Here's how the part is built. I have some questions about the finished solid (model axes, mm). Face numbers are marked on the shaded views. A direction names the side the tool comes from. Coordinates: 2 decimals unless noted, no trailing zeros. Write each loop counter-clockwise with the first axis right and the second up, starting at its lowest first coordinate (ties: lowest second). Pieces come first, ordered by that corner, then holes.
(1) Imagine slicing it at B-B, the plane y = -1. List the corners of the cut face in (x, z) for me, plus the area to 3 significant figures.
(2) Please list where these lines run through material, in increasing order: probe 1 along Z at (x, y) = (1.25, -2.25); probe 2 along X at (y, z) = (-1, -1); probe 3 along Y at (x, z) = (2.5, -32.5).
(3) Imagine slicing it at C-C, the plane z = -30. List the corners of the cut face in (x, y) for me.
(4) Imagine slicing it at A-A, the plane x = 0. List the corners of the cut face in (y, z) for me.
(5) Imagine slicing it at D-D, the plane x = -2.25. List the corners of the cut face in (y, z) for me.
(6) Which directions (+Z, -Z, +X, -X, +Y, -Y) give clear straight access to the entire face, cutting with the end or side of a thin tool? Please do the marked faces 1, 2 and 3.
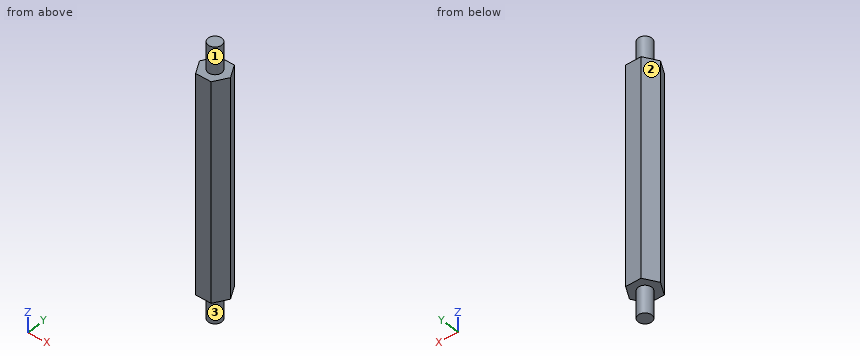
```python
from build123d import *

# Parameters (mm, degrees)
SM_BASE_FLANGE_1_DEPTH = 48
SKETCH_6_R             = 1.5
EXTRUDE_1_DEPTH        = 6
EXTRUDE_START          = 6
SKETCH_7_R             = 1.5
EXTRUDE_2_DEPTH        = 6


# Sheet-metal steps are written as plain solids
with BuildPart() as part:
    # Sketch 1 → 基体-法兰1 (new body)
    with BuildSketch(Plane.XY):
        Polygon((3.464101615, 0), (1.732050808, 3), (-1.732050808, 3), (-3.464101615, 0), (-1.732050808, -3), (1.732050808, -3), align=None)
    extrude(amount=-SM_BASE_FLANGE_1_DEPTH)

    # 草图6 → 凸台-拉伸1 (add)
    with BuildSketch(Plane.XY):
        Circle(SKETCH_6_R)
    extrude(amount=EXTRUDE_1_DEPTH)

    # 草图7 → 凸台-拉伸2 (add)
    with BuildSketch(Plane(origin=(0, 0, -48), x_dir=(-1, 0, 0), z_dir=(0, 0, -1)).offset(EXTRUDE_START)):
        with Locations(Location((0, 0, 0), (0, 0, 180))):
            Circle(SKETCH_7_R)
    extrude(amount=-EXTRUDE_2_DEPTH)


solid = part.part
```
Recorded:
1. outline: (-2.89, -48) - (-1.12, -48) - (-1.12, -54) - (1.12, -54) - (1.12, -48) - (2.89, -48) - (2.89, 0) - (1.12, 0) - (1.12, 6) - (-1.12, 6) - (-1.12, 0) - (-2.89, 0) - close
1. area: 304 mm2
2. probe 1: z = -48 to 0
2. probe 2: x = -2.89 to 2.89
2. probe 3: y = -1.67 to 1.67
3. outline: (-3.46, 0) - (-1.73, -3) - (1.73, -3) - (3.46, 0) - (1.73, 3) - (-1.73, 3) - close
4. outline: (-3, -48) - (-1.5, -48) - (-1.5, -54) - (1.5, -54) - (1.5, -48) - (3, -48) - (3, 0) - (1.5, 0) - (1.5, 6) - (-1.5, 6) - (-1.5, 0) - (-3, 0) - close
5. outline: (-2.1, -48) - (2.1, -48) - (2.1, 0) - (-2.1, 0) - close
6. face 1: +Z
6. face 2: +Z, -Z, -X, +Y
6. face 3: -Z
